from build123d import *

# Parameters (mm, degrees)
BASE_FLANGE1_DEPTH          = 110
CHAMFER1_SIZE2              = 3
CHAMFER1_SIZE               = 1.5
F_3_0MM_PRESS_DOWEL_HOLE1_D = 3


# Sheet-metal steps are written as plain solids
with BuildPart() as part:
    # Sketch1 → Base-Flange1 (new body)
    with BuildSketch(Plane(origin=(0, 0, 0), x_dir=(1, 0, 0), z_dir=(0, 1, 0))):
        with BuildLine():
            Line((0, 0), (0, -20))
            Line((0, -20), (0, -33.90302477))
            ThreePointArc((0, -33.90302477), (0.006301715, -33.999170363), (0.025099036, -34.093670879))
            Line((0.025099036, -34.093670879), (7.221834227, -60.952252257))
            ThreePointArc((7.221834227, -60.952252257), (7.252805527, -61.043490765), (7.295420878, -61.129906149))
            Line((7.295420878, -61.129906149), (21.198445648, -85.21065143))
            ThreePointArc((21.198445648, -85.21065143), (21.25197589, -85.290765098), (21.315505105, -85.363206285))
            Line((21.315505105, -85.363206285), (40.977351294, -105.025052473))
            ThreePointArc((40.977351294, -105.025052473), (41.04979248, -105.088581688), (41.129906149, -105.14211193))
            Line((41.129906149, -105.14211193), (65.21065143, -119.0451367))
            ThreePointArc((65.21065143, -119.0451367), (65.297066813, -119.087752052), (65.388305321, -119.118723352))
            Line((65.388305321, -119.118723352), (92.246886699, -126.315458542))
            ThreePointArc((92.246886699, -126.315458542), (92.341387215, -126.334255863), (92.437532808, -126.340557578))
            Line((92.437532808, -126.340557578), (106.340557578, -126.340557578))
            Line((106.340557578, -126.340557578), (106.340557578, -127.840557578))
            Line((106.340557578, -127.840557578), (92.437532808, -127.840557578))
            ThreePointArc((92.437532808, -127.840557578), (92.145597926, -127.821423155), (91.858658132, -127.764347281))
            Line((91.858658132, -127.764347281), (65.000076753, -120.567612091))
            ThreePointArc((65.000076753, -120.567612091), (64.723041665, -120.47357135), (64.46065143, -120.344174806))
            Line((64.46065143, -120.344174806), (40.379906149, -106.441150036))
            ThreePointArc((40.379906148, -106.441150036), (40.136650336, -106.278611699), (39.916691122, -106.085712644))
            Line((39.916691122, -106.085712645), (20.254844934, -86.423866456))
            ThreePointArc((20.254844934, -86.423866456), (20.06194588, -86.203907242), (19.899407542, -85.96065143))
            Line((19.899407542, -85.96065143), (5.996382772, -61.879906149))
            ThreePointArc((5.996382772, -61.879906149), (5.866986228, -61.617515913), (5.772945487, -61.340480825))
            Line((5.772945487, -61.340480825), (-1.423789703, -34.481899447))
            ThreePointArc((-1.423789703, -34.481899447), (-1.480865577, -34.194959652), (-1.5, -33.90302477))
            Line((-1.5, -33.90302477), (-1.5, -20))
            Line((-1.5, -20), (-1.5, 0))
            Line((-1.5, 0), (0, 0))
        make_face()
    extrude(amount=BASE_FLANGE1_DEPTH)

    # Chamfer1
    chamfer1_edges = [part.edges().sort_by_distance(p)[0] for p in [
        (106.340557578, 55, 126.340557578),
    ]]
    chamfer1_side = [part.faces().sort_by_distance(p)[0] for p in [
        (106.340557578, 55, 126.370557578),
    ]]
    chamfer(chamfer1_edges, length=CHAMFER1_SIZE - 0.0001, length2=CHAMFER1_SIZE2 - 0.0001, reference=chamfer1_side[0])  # a hair under: the kernel refuses the full size

    # Ø3.0mm Press Dowel Hole1 (through all)
    with Locations(Plane(origin=(-3, -55.405236378, -125.638352017), x_dir=(0, 0, 1), z_dir=(-1, 0, 0))):
        with Locations((154.541376787, 155.405236378), (154.541376787, 65.405236378)):
            Hole(F_3_0MM_PRESS_DOWEL_HOLE1_D / 2)


solid = part.part
Verification items for the finished model (mm, model axes). A direction names the side the tool comes from. Coordinates: 2 decimals unless noted, no trailing zeros. Loops run counter-clockwise (first coordinate to the right, second up) from the corner with the lowest first, then second, coordinate; pieces in that order, holes last. Notation, with made-up numbers: (-31.75, 7) -> (25.25, 7) arc R20 cw to (25.25, 41) -> close; hole circle Ø10 at (51.5, 37). An arc over 180 degrees is marked (long way). Write each question's results on one line, items separated by ' | '.
Item 1: Section check B-B, the plane x = 60.5. Enter the section's corners in (y, z).
Found:
outline: (0, 116.33) -> (110, 116.33) -> (110, 118.06) -> (0, 118.06) -> close
Item 2: Section check C-C, the plane z = 41. Enter the section's corners in (x, y), plus the area to 3 significant figures.
Found:
outline: (0.32, 0) -> (1.88, 0) -> (1.88, 110) -> (0.32, 110) -> close | area: 171 mm2
Item 3: Gauge pin test, flat ends, axial feed: pin 1 (3.5 mm diameter, centred on x = 98.5, y = 37, fed in from -Z); pin 2 (3 mm diameter, centred on y = 81, z = 57.5, fed in from +X); pin 3 (12 mm diameter, centred on y = 64, z = 36.5, fed in from +X). Record the tip position at first contact, or that the pin passes through.
Found:
pin 1: stops at z = 126.34 | pin 2: stops at x = 6.7 | pin 3: stops at x = 2.28
Item 4: Tool access check on faces 1 (the face through (-1.5, 54, 17)), 2 (the face through (0, 54, 17)). Record the directions out of +Z, -Z, +X, -X, +Y, -Y that give a thin tool (end or side, any length) a straight path to the whole face; none if there is none.
Found:
face 1: +Z, -Z, -X, +Y, -Y | face 2: -Z, +X, +Y, -Y
Item 5: Material ranges on L1, parallel to X at y = 74, z = 26; L2, parallel to X at y = 96, z = 87.5; L3, parallel to Z at x = 18, y = 37.5, recorded low to high.
Found:
L1: x = -1.5 to 0 | L2: x = 21.33 to 23.45 | L3: z = 79.67 to 82.67
